Check sheet for the drawn part. Datum: minimum x, y, z corner. Units: mm. A direction names the side the tool comes from. Give positions to 0.01 mm unless a question says otherwise; leave off trailing zeros. Order: outer loops, then holes, each group sorted by start corner. A loop starts at its lowest first (then second) coordinate and runs counter-clockwise, first axis right, second up.
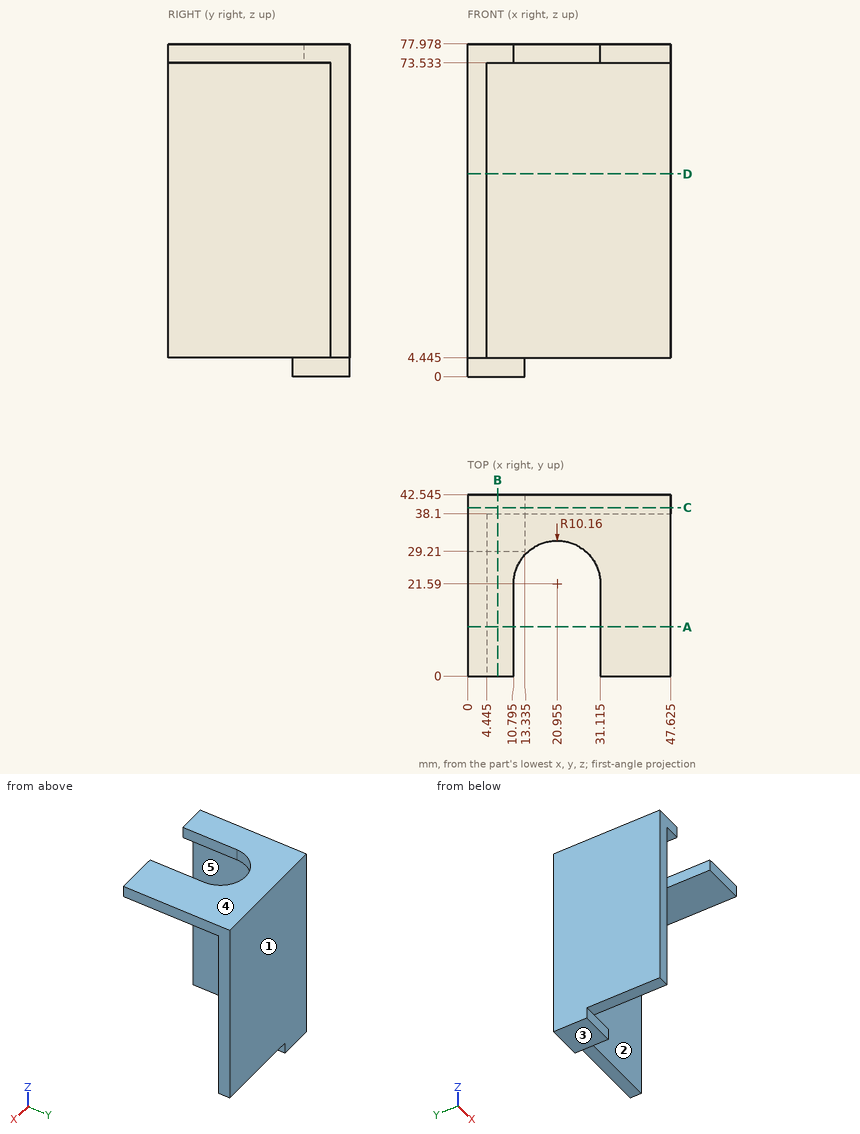
Item 1: Sectioned sample at B-B (x = 7). Enter the section's corners in (y, z) (3 decimals), and give its area (3 significant figures).
Reported:
outline: (0, 73.533) - (38.1, 73.533) - (38.1, 4.445) - (29.21, 4.445) - (29.21, 0) - (42.545, 0) - (42.545, 77.978) - (0, 77.978) - close
area: 555 mm2
Item 2: Sectioned sample at D-D (z = 47.5). Enter the section's corners in (x, y) (3 decimals).
Reported:
outline: (0, 0) - (4.445, 0) - (4.445, 38.1) - (47.625, 38.1) - (47.625, 42.545) - (0, 42.545) - close
Item 3: Draft check along Z on the marked faces 1, 2 and 3. Enter one of: released by +Z, released by -Z, zero draft, split by the parting line, or undercut.
Reported:
face 1: zero draft
face 2: undercut
face 3: released by -Z
Item 4: Sectioned sample at A-A (y = 11.5). Enter the section's corners in (x, z) (3 decimals).
Reported:
outline: (0, 4.445) - (4.445, 4.445) - (4.445, 73.533) - (10.795, 73.533) - (10.795, 77.978) - (0, 77.978) - close; (31.115, 73.533) - (47.625, 73.533) - (47.625, 77.978) - (31.115, 77.978) - close
Item 5: Gauge pin test, flat ends, axial feed: pin 1 (3.5 mm diameter, centred on y = 10.5, z = 75, fed in from -X); pin 2 (3.5 mm diameter, centred on x = 6.5, z = 2.5, fed in from -Y); pin 3 (11.5 mm diameter, centred on y = 18.5, z = 33, fed in from +X) (3 decimals); pin 4 (5 mm diameter, centred on x = 36, y = 40, fed in from -Z) (3 decimals). Record the tip position at first contact, or that the pin passes through.
Reported:
pin 1: stops at x = 0
pin 2: stops at y = 29.21
pin 3: stops at x = 4.445
pin 4: stops at z = 4.445
Item 6: Set-up check for the marked faces 4 and 5: record each of +Z, -Z, +X, -X, +Y, -Y from which the full face is reachable in a straight line by a thin tool's end or side.
Reported:
face 4: +Z, +X, -X, +Y, -Y
face 5: +X, -Y
Item 7: Scan lines: L1, parallel to Z at x = 12, y = 37.5 (3 decimals); L2, parallel to Y at x = 6.5, z = 67 (3 decimals); L3, parallel to X at y = 16, z = 40.5 (3 decimals). Record each from-to range of solid material in increasing order.
Reported:
L1: z = 0 to 4.445, 73.533 to 77.978
L2: y = 38.1 to 42.545
L3: x = 0 to 4.445
Item 8: Sectioned sample at C-C (y = 39.5). Enter the section's corners in (x, z) (3 decimals), and give its area (3 significant figures).
Reported:
outline: (0, 0) - (13.335, 0) - (13.335, 4.445) - (47.625, 4.445) - (47.625, 77.978) - (0, 77.978) - close
area: 3,560 mm2
